Verification items for the finished model (mm, model axes). A direction names the side the tool comes from. Give positions to 0.01 mm unless a question says otherwise; leave off trailing zeros. Order: outer loops, then holes, each group sorted by start corner. A loop starts at its lowest first (then second) coordinate and runs counter-clockwise, first axis right, second up.
from build123d import *

# Parameters (mm, degrees)
F1_DEPTH = 965.2
F2_R     = 5.08
F4_DEPTH = 76.2


with BuildPart() as f1:
    # F0 (on Front) → F1 (new body, symmetric)
    with BuildSketch(Plane.XZ):
        Polygon((-38.1, -38.1), (38.1, -38.1), (38.1, -31.75), (-31.75, -31.75), (-31.75, 38.1), (-38.1, 38.1), align=None)
    extrude(amount=F1_DEPTH, both=True)

    # F2
    f2_edges = [f1.edges().sort_by_distance(p)[0] for p in [
        (-31.75, 0, 38.1),
        (-31.75, 0, -31.75),
        (38.1, 0, -31.75),
    ]]
    fillet(f2_edges, radius=F2_R)

    # F3 (on face) → F4 (cut)
    with BuildSketch(Plane(origin=(-38.1, 0, 0), x_dir=(0, -1, 0), z_dir=(-1, 0, 0))):
        Polygon((-965.2, 38.1), (-965.2, -38.1), (-889, 38.1), align=None)
        Polygon((889, 38.1), (965.2, -38.1), (965.2, 38.1), align=None)
    extrude(amount=-F4_DEPTH, mode=Mode.SUBTRACT)


solid = f1.part
(1) Section check C-C, the plane x = 6. Enter the section's corners in (y, z), then the cut area to 3 significant figures.
Solved:
outline: (-965.2, -38.1) - (965.2, -38.1) - (958.85, -31.75) - (-958.85, -31.75) - close
area: 12,200 mm2
(2) Section check B-B, the plane z = 2. Enter the section's corners in (x, y), then the cut area to 3 significant figures.
Solved:
outline: (-38.1, -925.1) - (-31.75, -925.1) - (-31.75, 925.1) - (-38.1, 925.1) - close
area: 11,700 mm2
(3) Section check A-A, the plane y = 294. Enter the section's corners in (x, z), then the cut area to 3 significant figures.
Solved:
outline: (-38.1, -38.1) - (38.1, -38.1) - (38.1, -36.83) arc R5.08 ccw to (33.02, -31.75) - (-26.67, -31.75) arc R5.08 cw to (-31.75, -26.67) - (-31.75, 33.02) arc R5.08 ccw to (-36.83, 38.1) - (-38.1, 38.1) - close
area: 922 mm2
(4) Set-up check for faces 4 (the flat face through (-1, -14, -38.1)), 5 (the flat face through (4, -13, -31.75)): record each of +Z, -Z, +X, -X, +Y, -Y from which the full face is reachable in a straight line by a thin tool's end or side.
Solved:
face 4: -Z, +X, -X, +Y, -Y
face 5: +Z, +X, +Y, -Y
(5) Go/stop test with flat-tipped pins: pin 1 (5 mm diameter, centred on x = 15.5, y = -200, fed in from +Z); pin 2 (4 mm diameter, centred on y = -620.5, z = 10, fed in from +X). Record where each tip stops, or that it passes through.
Solved:
pin 1: stops at z = -31.75
pin 2: stops at x = -31.75
(6) Release check for a two-part mould opening along X. For faces 1 (the flat face through (-38.1, -14, 1)), 2 (the flat face through (-31.75, -13, 3)), 3 (the flat face through (-34, -943.9, -16.8)) record: pulls with the +X half, pulls with the -X half, needs draft (parallel to the pull), parting line crosses it, or undercut.
Solved:
face 1: pulls with the -X half
face 2: pulls with the +X half
face 3: needs draft
(7) Scan lines: line 1 (Z direction, x = 17, y = 806.5); line 2 (X direction, y = -563, z = -28). Record each from-to range of solid material in increasing order.
Solved:
line 1: z = -38.1 to -31.75
line 2: x = -38.1 to -31.57
